Autodesk Inventor part; units mm, degrees
ref_plane "YZ Plane" through (0, 0, 0) normal (1, 0, 0) x (0, 1, 0)
ref_plane "XZ Plane" through (0, 0, 0) normal (0, 1, 0) x (-1, 0, 0)
ref_plane "XY Plane" through (0, 0, 0) normal (0, 0, 1) x (1, 0, 0)
sketch "Skizze1" plane through (0, 0, 0) normal (0, 0, 1) x (1, 0, 0)
  line L0 (-10, -30.5) -> (10, -30.5)
  line L1 (10, -30.5) -> (10, 30.5)
  line L2 (10, 30.5) -> (-10, 30.5)
  line L3 (-10, 30.5) -> (-10, -30.5)
  line L4 (-10, -30.5) -> (10, 30.5) construction
  line L5 (10, -30.5) -> (-10, 30.5) construction
  point P0 (0, 0)
  dimension "d0" = 20
  dimension "d1" = 61
extrude "Extrusion1" add sketch "Skizze1" along normal blind 2
sketch "Skizze3" plane through (0, 0, 0) normal (0, 0, -1) x (-1, 0, 0)
  line L0 (10, 30.5) -> (10, -30.5)
  line L1 (-10, -20.5) -> (10, -20.5)
  line L2 (10, -20.5) -> (10, 20.5)
  line L3 (10, 20.5) -> (-10, 20.5)
  line L4 (-10, 20.5) -> (-10, -20.5)
  line L5 (-10, -20.5) -> (10, 20.5) construction
  line L6 (10, -20.5) -> (-10, 20.5) construction
  line L7 (10, -30.5) -> (-10, -30.5)
  line L8 (-10, -30.5) -> (-10, 30.5)
  point P0 (0, 0)
  point P1 (10, -20.5)
  dimension "d9" = 41
  dimension "d17" = 10
extrude "Extrusion3" add sketch "Skizze3" along normal blind 13 contours L0 L1 L4 L3
sketch "Skizze4" plane through (-10, -30.5, 2) normal (-1, 0, 0) x (0, 0, 1)
  line L0 (-2, 10) -> (-15, 10)
  line L1 (-12.32, 10) -> (-2, 10)
  line L2 (-2, 10) -> (-2, 11.25)
  line L3 (-2, 11.25) -> (-12.32, 11.25)
  line L4 (-12.32, 11.25) -> (-12.32, 10)
  line L5 (-15, 10) -> (-15, 51)
  line L6 (-4.404, 30.5) -> (2.981, 30.5) construction
  line L7 (-2, 51) -> (-15, 51)
  line L8 (-2, 51) -> (-2, 49.75)
  line L9 (-2, 49.75) -> (-12.32, 49.75)
  line L10 (-12.32, 49.75) -> (-12.32, 51)
  line L11 (-2, 10) -> (-12.32, 10)
  point P0 (-2, 30.5)
  point P1 (-12.32, 10.625)
  dimension "d12" = 2.68
  dimension "d13" = 1.25
extrude "Extrusion4" cut sketch "Skizze4" against normal through all
fillet "Rundung1" radius 1 6 edges at (-10, -30.5, 1) (10, -30.5, 1) (10, 30.5, 1) (-10, 30.5, 1) (0, 20.5, -13) (0, -20.5, -13)
sketch "Skizze6" plane through (0, 0, 2) normal (0, 0, 1) x (1, 0, 0)
  point P0 (0, 0)
sketch "Skizze7" plane through (0, 0, 2) normal (0, 0, 1) x (1, 0, 0)
  line L0 (-8.9, 11.275) -> (8.9, 11.275)
  line L1 (8.9, 11.275) -> (8.9, -11.275)
  line L2 (8.9, -11.275) -> (-8.9, -11.275)
  line L3 (-8.9, -11.275) -> (-8.9, 11.275)
  line L4 (-8.9, 11.275) -> (8.9, -11.275) construction
  line L5 (8.9, 11.275) -> (-8.9, -11.275) construction
  line L6 (-8.9, 11.275) -> (-10, 11.275)
  line L7 (-10, 11.275) -> (-10, -11.275)
  line L8 (-10, -11.275) -> (-8.9, -11.275)
  line L9 (8.9, 11.275) -> (10, 11.275)
  line L10 (10, 11.275) -> (10, -11.275)
  line L11 (10, -11.275) -> (8.9, -11.275)
  line L12 (10, -29.5) -> (10, 29.5)
  line L13 (-10, 29.5) -> (-10, -29.5)
  line L14 (-3.1, 12.775) -> (3.1, 12.775)
  line L15 (3.1, 12.775) -> (3.1, 11.275)
  line L16 (3.1, 11.275) -> (-3.1, 11.275)
  line L17 (-3.1, 11.275) -> (-3.1, 12.775)
  line L18 (-3.1, 12.775) -> (3.1, 11.275) construction
  line L19 (3.1, 12.775) -> (-3.1, 11.275) construction
  line L20 (-0.8378, 0) -> (1.8317, 0) construction
  line L21 (-3.1, -12.775) -> (3.1, -12.775)
  line L22 (3.1, -12.775) -> (3.1, -11.275)
  line L23 (3.1, -11.275) -> (-3.1, -11.275)
  line L24 (-3.1, -11.275) -> (-3.1, -12.775)
  line L25 (10, 11.275) -> (8.9, 11.275)
  line L26 (8.9, 11.275) -> (8.9, 26.275)
  line L27 (8.9, 26.275) -> (10, 26.275)
  line L28 (10, 26.275) -> (10, 11.275)
  line L29 (0, 1.7909) -> (0, -1.8992) construction
  line L30 (8.9, -11.275) -> (10, -11.275)
  line L31 (10, 29.5) -> (10, -29.5)
  line L32 (8.9, -11.275) -> (8.9, -26.275)
  line L33 (8.9, -26.275) -> (10, -26.275)
  line L34 (-8.9, 11.275) -> (-10, 11.275)
  line L35 (-10, -11.275) -> (-8.9, -11.275)
  line L36 (-10, -29.5) -> (-10, 29.5)
  line L37 (-8.9, 11.275) -> (-8.9, 26.275)
  line L38 (-8.9, 26.275) -> (-10, 26.275)
  line L39 (-8.9, -11.275) -> (-8.9, -26.275)
  line L40 (-8.9, -26.275) -> (-10, -26.275)
  point P0 (0, 0)
  point P1 (0, 0)
  point P2 (0, 12.025)
  point P3 (8.9, 18.775)
  dimension "d36" = 17.8
  dimension "d37" = 22.55
  dimension "d38" = 6.2
  dimension "d39" = 1.5
  dimension "d45" = 15
extrude "Extrusion5" add sketch "Skizze7" along normal blind 7 contours L3 L8 L7 L6 | L6 L13 L38 L37 | L17 L14 L15 L0 | L39 L40 L13 L8 | L2 L22 L21 L24 | L9 L10 L11 L1 | L26 L27 L12 L9 | L11 L12 L33 L32
chamfer "Fasen1" distance 2 angle 45 2 edges at (0, -19.25, 0) (0, 19.25, 0)
chamfer "Fasen2" distance 3 angle 45 2 edges at (0, 12.775, 2) (0, -12.775, 2)
chamfer "Fasen3" distance 2.5 angle 45 4 edges at (9.45, -26.275, 2) (-9.45, -26.275, 2) (-9.45, 26.275, 2) (9.45, 26.275, 2)
sketch "Skizze8" plane through (0, 0, 2) normal (0, 0, 1) x (1, 0, 0)
  circle A0 centre (0, 25.5) radius 2.5
  line L0 (1.3354, 0) -> (-2.5, 0) construction
  circle A1 centre (0, -25.5) radius 2.5
  line L1 (9, 30.5) -> (-9, 30.5)
  point P0 (0, 0)
  point P1 (0, 30.5)
  dimension "d52" = 5
  dimension "d55" = 5
extrude "Extrusion6" cut sketch "Skizze8" against normal through all
fillet "Rundung2" radius 1 4 edges at (-9.45, -26.275, 9) (9.45, -26.275, 9) (-9.45, 26.275, 9) (9.45, 26.275, 9)
fillet "Rundung3" radius 0.5 2 edges at (-8.9, 0, 2) (8.9, 0, 2)
fillet "Rundung4" radius 0.5 2 edges at (0, -11.275, 2) (0, 11.275, 2)
properties part number "Relais_Platte_3D-Druck"
Input: part model. Units: mm. Frame: model coordinates. A direction names the side the tool comes from. Round coordinates to 2 decimals unless told otherwise and drop trailing zeros. Loops run counter-clockwise (first coordinate to the right, second up) from the corner with the lowest first, then second, coordinate; pieces in that order, holes last.
1) Material intervals for line 1 (Y direction, x = 0, z = 1.2); line 2 (X direction, y = -25, z = 5.5); line 3 (Z direction, x = 0, y = 8), sorted ascending.
Ans:
line 1: y = -30.5 to -28, -23 to 23, 28 to 30.5
line 2: x = -10 to -8.9, 8.9 to 10
line 3: z = -13 to 2
2) Set-up query: faces 5 (the flat face through (0, 0, 2)), 6 (the flat face through (-0.043, 14.254, 3.521)), 7 (the flat face through (0, -12.775, 7)), 8 (the flat face through (-3.1, 12.7, 4.7)), 9 (the flat face through (-9.4, 26.275, 6.2)). Return all of +Z, -Z, +X, -X, +Y, -Y with unobstructed straight access to the full face (end or side cutting, diameter ignored); none if empty.
Ans:
face 5: +Z
face 6: +Z, +Y
face 7: +Z, -Y
face 8: +Z, +Y, -Y
face 9: +Z, +X, -X, +Y
3) Pin query (flat end, axial travel): pin 1 (6 mm diameter, centred on x = -5, z = -8.5, fed in from +Y); pin 2 (3 mm diameter, centred on x = 0, z = 7.5, fed in from +Y) (3 decimals); pin 3 (2 mm diameter, centred on x = -6, y = 10.5, fed in from +Z). Return the tip coordinate at first contact, or that it passes through.
Ans:
pin 1: stops at y = 20.5
pin 2: stops at y = 12.775
pin 3: stops at z = 2
4) Pull-direction query (Z, two-part tool) for faces 1 (the flat face through (0, -19.25, -6)), 2 (the flat face through (0, 12.775, 7)), 3 (the flat face through (-9.367, -27.508, 3.267)), 4 (the flat face through (0, 0, -13)); classes: released by +Z, released by -Z, zero draft, split by the parting line, or undercut.
Ans:
face 1: undercut
face 2: zero draft
face 3: released by +Z
face 4: released by -Z
5) Section query D-D on x = 0. Count the separate pieces of the cut face and the enclosed holes in it, plus the area to 3 significant figures.
Ans:
separate pieces: 3
enclosed holes: 0
area: 643 mm2
6) Section query B-B on y = -16.5. Return the cut outline in (x, z), plus the area to 3 significant figures.
Ans:
outline: (-10, -13) - (10, -13) - (10, 9) - (8.9, 9) - (8.9, 2.5) arc R0.5 cw to (8.4, 2) - (-8.4, 2) arc R0.5 cw to (-8.9, 2.5) - (-8.9, 9) - (-10, 9) - close
area: 316 mm2
7) Section query A-A on x = -7.75. Return the cut outline in (y, z).
Ans:
outline: (-30.5, 0) - (-21.25, 0) - (-19.25, -2) - (-19.25, -10.32) - (-20.5, -10.32) - (-20.5, -12) arc R1 ccw to (-19.5, -13) - (19.5, -13) arc R1 ccw to (20.5, -12) - (20.5, -10.32) - (19.25, -10.32) - (19.25, -2) - (21.25, 0) - (30.5, 0) - (30.5, 2) - (-30.5, 2) - close
8) Section query C-C on z = -7. Return the cut outline in (x, y), plus the area to 3 significant figures.
Ans:
outline: (-10, -19.25) - (10, -19.25) - (10, 19.25) - (-10, 19.25) - close
area: 770 mm2
